Could you check a few things on this model? Use its own coordinates, in mm. A direction names the side the tool comes from. Round coordinates to 2 decimals unless told otherwise and drop trailing zeros. Loops run counter-clockwise (first coordinate to the right, second up) from the corner with the lowest first, then second, coordinate; pieces in that order, holes last. Notation, with made-up numbers: (84, 41) - (129, 41) arc R19 cw to (129, 48) - close; hole circle Ø3 at (-20, -1). An arc over 180 degrees is marked (long way). Put each result on its own line as item: value. Start each with the question number.
from build123d import *

# Parameters (mm, degrees)
BOSS_EXTRU_1_DEPTH      = 42
ESQUISSE3_R             = 19.05
BOSS_EXTRU_2_DEPTH      = 1.6
CHANFREIN1_SIZE         = 0.2
CONG_1_R                = 0.2
ESQUISSE4_R             = 3.175
BOSS_EXTRU_3_DEPTH      = 5.6
BOSS_EXTRU_4_DEPTH      = 15
CHANFREIN2_SIZE         = 0.4
ENL_V_START             = -37
ENL_V_MAT_EXTRU_1_DEPTH = 37
ENL_V_MAT_EXTRU_2_DEPTH = 59.210823736


with BuildPart() as part:
    # Esquisse1 → Boss.-Extru.1 (new body)
    with BuildSketch(Plane.XY):
        with BuildLine():
            Line((-26.5, -28.5), (26.5, -28.5))
            ThreePointArc((26.5, -28.5), (27.914213562, -27.914213562), (28.5, -26.5))
            Line((28.5, -26.5), (28.5, 26.5))
            ThreePointArc((28.5, 26.5), (27.914213562, 27.914213562), (26.5, 28.5))
            Line((26.5, 28.5), (-26.5, 28.5))
            ThreePointArc((-26.5, 28.5), (-27.914213562, 27.914213562), (-28.5, 26.5))
            Line((-28.5, 26.5), (-28.5, -26.5))
            ThreePointArc((-28.5, -26.5), (-27.914213562, -27.914213562), (-26.5, -28.5))
        make_face()
    extrude(amount=-BOSS_EXTRU_1_DEPTH)

    # Esquisse3 → Boss.-Extru.2 (add)
    with BuildSketch(Plane.XY):
        Circle(ESQUISSE3_R)
    extrude(amount=BOSS_EXTRU_2_DEPTH)

    # Chanfrein1
    chanfrein1_edges = [part.edges().sort_by_distance(p)[0] for p in [
        (-19.05, 0, 1.6),
    ]]
    chamfer(chanfrein1_edges, length=CHANFREIN1_SIZE)

    # Congé1
    cong_1_edges = [part.edges().sort_by_distance(p)[0] for p in [
        (-19.05, 0, 0),
    ]]
    fillet(cong_1_edges, radius=CONG_1_R)

    # Esquisse4 → Boss.-Extru.3 (add)
    with BuildSketch(Plane.XY.offset(1.6)):
        Circle(ESQUISSE4_R)
    extrude(amount=BOSS_EXTRU_3_DEPTH)

    # Esquisse5 → Boss.-Extru.4 (add)
    with BuildSketch(Plane.XY.offset(7.2)):
        with BuildLine():
            Line((-1.710263138, 2.675), (1.710263138, 2.675))
            ThreePointArc((1.710263138, 2.675), (0, -3.175), (-1.710263138, 2.675))
        make_face()
    extrude(amount=BOSS_EXTRU_4_DEPTH)

    # Chanfrein2
    chanfrein2_edges = [part.edges().sort_by_distance(p)[0] for p in [
        (0, -3.175, 22.2),
        (0, 2.675, 22.2),
    ]]
    chamfer(chanfrein2_edges, length=CHANFREIN2_SIZE)

    # Esquisse7 → Enlèv. mat.-Extru.1 (cut)
    with BuildSketch(Plane(origin=(0, 0, -42), x_dir=(-1, 0, 0), z_dir=(0, 0, -1)).offset(ENL_V_START)):
        with BuildLine():
            Line((-28.5, 26.5), (-28.5, 16.5))
            ThreePointArc((-28.5, 16.5), (-27.914213562, 17.914213562), (-26.5, 18.5))
            Line((-26.5, 18.5), (-23.5, 18.5))
            ThreePointArc((-23.5, 18.5), (-19.964466094, 19.964466094), (-18.5, 23.5))
            Line((-18.5, 23.5), (-18.5, 26.5))
            ThreePointArc((-18.5, 26.5), (-17.914213562, 27.914213562), (-16.5, 28.5))
            Line((-16.5, 28.5), (-26.5, 28.5))
            ThreePointArc((-26.5, 28.5), (-27.914213562, 27.914213562), (-28.5, 26.5))
        make_face()
        with BuildLine():
            Line((26.5, 28.5), (16.5, 28.5))
            ThreePointArc((16.5, 28.5), (17.914213562, 27.914213562), (18.5, 26.5))
            Line((18.5, 26.5), (18.5, 23.5))
            ThreePointArc((18.5, 23.5), (19.964466094, 19.964466094), (23.5, 18.5))
            Line((23.5, 18.5), (26.5, 18.5))
            ThreePointArc((26.5, 18.5), (27.914213562, 17.914213562), (28.5, 16.5))
            Line((28.5, 16.5), (28.5, 26.5))
            ThreePointArc((28.5, 26.5), (27.914213562, 27.914213562), (26.5, 28.5))
        make_face()
        with BuildLine():
            ThreePointArc((18.5, -26.5), (17.914213562, -27.914213562), (16.5, -28.5))
            Line((16.5, -28.5), (26.5, -28.5))
            ThreePointArc((26.5, -28.5), (27.914213562, -27.914213562), (28.5, -26.5))
            Line((28.5, -26.5), (28.5, -16.5))
            ThreePointArc((28.5, -16.5), (27.914213562, -17.914213562), (26.5, -18.5))
            Line((26.5, -18.5), (23.5, -18.5))
            ThreePointArc((23.5, -18.5), (19.964466094, -19.964466094), (18.5, -23.5))
            Line((18.5, -23.5), (18.5, -26.5))
        make_face()
        with BuildLine():
            ThreePointArc((-18.5, -23.5), (-19.964466094, -19.964466094), (-23.5, -18.5))
            Line((-23.5, -18.5), (-26.5, -18.5))
            ThreePointArc((-26.5, -18.5), (-27.914213562, -17.914213562), (-28.5, -16.5))
            Line((-28.5, -16.5), (-28.5, -26.5))
            ThreePointArc((-28.5, -26.5), (-27.914213562, -27.914213562), (-26.5, -28.5))
            Line((-26.5, -28.5), (-16.5, -28.5))
            ThreePointArc((-16.5, -28.5), (-17.914213562, -27.914213562), (-18.5, -26.5))
            Line((-18.5, -26.5), (-18.5, -23.5))
        make_face()
    extrude(amount=ENL_V_MAT_EXTRU_1_DEPTH, mode=Mode.SUBTRACT)

    # Esquisse6 → Enlèv. mat.-Extru.2 (cut, through all)
    with BuildSketch(Plane.XY):
        with BuildLine():
            Line((-23.5, 20.95), (-23.5, 23.5))
            Line((-23.5, 23.5), (-20.95, 23.5))
            ThreePointArc((-20.95, 23.5), (-25.303122292, 25.303122292), (-23.5, 20.95))
        make_face()
        with BuildLine():
            Line((-20.95, 23.5), (-23.5, 23.5))
            Line((-23.5, 23.5), (-23.5, 20.95))
            ThreePointArc((-23.5, 20.95), (-21.696877708, 21.696877708), (-20.95, 23.5))
        make_face()
        with BuildLine():
            ThreePointArc((26.05, 23.5), (23.5, 26.05), (20.95, 23.5))
            Line((20.95, 23.5), (23.5, 23.5))
            Line((23.5, 23.5), (23.5, 20.95))
            ThreePointArc((23.5, 20.95), (25.303122292, 21.696877708), (26.05, 23.5))
        make_face()
        with BuildLine():
            Line((23.5, 23.5), (20.95, 23.5))
            ThreePointArc((20.95, 23.5), (21.696877708, 21.696877708), (23.5, 20.95))
            Line((23.5, 20.95), (23.5, 23.5))
        make_face()
        with BuildLine():
            ThreePointArc((26.05, -23.5), (25.303122292, -21.696877708), (23.5, -20.95))
            Line((23.5, -20.95), (23.5, -23.5))
            Line((23.5, -23.5), (20.95, -23.5))
            ThreePointArc((20.95, -23.5), (23.5, -26.05), (26.05, -23.5))
        make_face()
        with BuildLine():
            Line((23.5, -23.5), (23.5, -20.95))
            ThreePointArc((23.5, -20.95), (21.696877708, -21.696877708), (20.95, -23.5))
            Line((20.95, -23.5), (23.5, -23.5))
        make_face()
        with BuildLine():
            ThreePointArc((-20.95, -23.5), (-21.696877708, -21.696877708), (-23.5, -20.95))
            Line((-23.5, -20.95), (-23.5, -23.5))
            Line((-23.5, -23.5), (-20.95, -23.5))
        make_face()
        with BuildLine():
            Line((-23.5, -23.5), (-23.5, -20.95))
            ThreePointArc((-23.5, -20.95), (-25.303122292, -25.303122292), (-20.95, -23.5))
            Line((-20.95, -23.5), (-23.5, -23.5))
        make_face()
    extrude(amount=-ENL_V_MAT_EXTRU_2_DEPTH, mode=Mode.SUBTRACT)


solid = part.part
Item 1: Will these pins go through, and if not, where does the flat tip stop? P1, Ø1, axis at x = -9, z = 1.5, coming from the +Y side; P2, Ø0.9, axis at x = -25, z = -22, coming from the -Y side; P3, Ø6.5, axis at x = -23.5, y = 23.5, coming from the -Z side.
Item 2: On a 3-axis mill with a long thin cutter (end or side, diameter ignored), from which of +Z, -Z, +X, -X, +Y, -Y can I reach the whole of each face in a straight line? I mean faces 1 (the face through (-15.12, -11.59, 0.79)), 2 (the face through (27.9, -17.93, -23.24)), 3 (the face through (27, 24, -5)), 4 (the face through (-17.9, 27.93, -23.24)). Say none if no direction works.
Item 3: Suppose I cut it at B-B, the plane x = -22. List the corners of the cut face in (y, z) for me.
Item 4: I need wall thicknesses on line 1 (Y direction, x = -23.5, z = -2.8); line 2 (Z direction, x = 19, y = 12). Which ranges of each line are inside material? Lowest first, please. Write a range as from..to.
Item 5: Suppose I cut it at C-C, the plane z = -18. List the corners of the cut face in (x, y) for me.
Item 6: Suppose I cut it at D-D, the plane x = 0. List the corners of the cut face in (y, z) for me (3 decimals), then the cut area to 3 significant figures.
Item 7: Suppose I cut it at A-A, the plane y = 0. List the corners of the cut face in (x, z) for me (3 decimals).
Numbers:
1. P1: y = 17.04
1. P2: y = -18.5
1. P3: z = -5
2. face 1: +Z
2. face 2: -Z, +X, -Y
2. face 3: -Z, +X, +Y
2. face 4: -Z, -X, +Y
3. outline: (-28.5, -5) - (-25.56, -5) - (-25.56, 0) - (-28.5, 0) - close; (-21.44, -5) - (-18.73, -5) - (-18.73, -42) - (18.73, -42) - (18.73, -5) - (21.44, -5) - (21.44, 0) - (-21.44, 0) - close; (25.56, -5) - (28.5, -5) - (28.5, 0) - (25.56, 0) - close
4. line 1: -28.5..-26.05, -20.95..20.95, 26.05..28.5
4. line 2: -42..0
5. outline: (-28.5, -16.5) arc R2 ccw to (-26.5, -18.5) - (-23.5, -18.5) arc R5 cw to (-18.5, -23.5) - (-18.5, -26.5) arc R2 ccw to (-16.5, -28.5) - (16.5, -28.5) arc R2 ccw to (18.5, -26.5) - (18.5, -23.5) arc R5 cw to (23.5, -18.5) - (26.5, -18.5) arc R2 ccw to (28.5, -16.5) - (28.5, 16.5) arc R2 ccw to (26.5, 18.5) - (23.5, 18.5) arc R5 cw to (18.5, 23.5) - (18.5, 26.5) arc R2 ccw to (16.5, 28.5) - (-16.5, 28.5) arc R2 ccw to (-18.5, 26.5) - (-18.5, 23.5) arc R5 cw to (-23.5, 18.5) - (-26.5, 18.5) arc R2 ccw to (-28.5, 16.5) - close
6. outline: (-28.5, -42) - (28.5, -42) - (28.5, 0) - (19.25, 0) arc R0.2 cw to (19.05, 0.2) - (19.05, 1.4) - (18.85, 1.6) - (3.175, 1.6) - (3.175, 7.2) - (2.675, 7.2) - (2.675, 21.8) - (2.275, 22.2) - (-2.775, 22.2) - (-3.175, 21.8) - (-3.175, 1.6) - (-18.85, 1.6) - (-19.05, 1.4) - (-19.05, 0.2) arc R0.2 cw to (-19.25, 0) - (-28.5, 0) - close
6. area: 2,580 mm^2
7. outline: (-28.5, -42) - (28.5, -42) - (28.5, 0) - (19.25, 0) arc R0.2 cw to (19.05, 0.2) - (19.05, 1.4) - (18.85, 1.6) - (3.175, 1.6) - (3.175, 21.8) - (2.775, 22.2) - (-2.775, 22.2) - (-3.175, 21.8) - (-3.175, 1.6) - (-18.85, 1.6) - (-19.05, 1.4) - (-19.05, 0.2) arc R0.2 cw to (-19.25, 0) - (-28.5, 0) - close
